Geometry: final body of the model. Coordinates: model frame, mm. Face numbers are marked on the shaded views. A direction names the side the tool comes from. Coordinates: 2 decimals unless noted, no trailing zeros. Loops run counter-clockwise (first coordinate to the right, second up) from the corner with the lowest first, then second, coordinate; pieces in that order, holes last. Notation, with made-up numbers: M -7.75,72.25 L 15.25,72.25 A18 ccw 15.25,83.25 Z; hole C 74.5,37.5 d2. An arc over 180 degrees is marked long. Write each question's results on one line, items separated by ' | '. Start each with the question number.
from build123d import *


with BuildPart() as part:
    # Sketch1 → Revolve3 (revolve)
    with BuildSketch(Plane.XY, mode=Mode.PRIVATE) as revolve3_sk:
        with BuildLine():
            Line((0, 0), (22.86, 0))
            Line((22.86, 0), (25.4, 2.54))
            Line((25.4, 2.54), (25.4, 8.89))
            Line((25.4, 8.89), (21.59, 12.7))
            Line((21.59, 12.7), (0, 12.7))
            Line((0, 12.7), (0, 11.43))
            Line((0, 11.43), (4.988818102, 8.549704526))
            ThreePointArc((4.988818102, 8.549704526), (6.258818102, 6.35), (4.988818102, 4.150295474))
            Line((4.988818102, 4.150295474), (0, 1.27))
            Line((0, 1.27), (0, 0))
        make_face()
    revolve(revolve3_sk.sketch.rotate(Axis((41.91, 0, 0), (0, 1, 0)), 270), axis=Axis((41.91, 0, 0), (0, 1, 0)))


solid = part.part
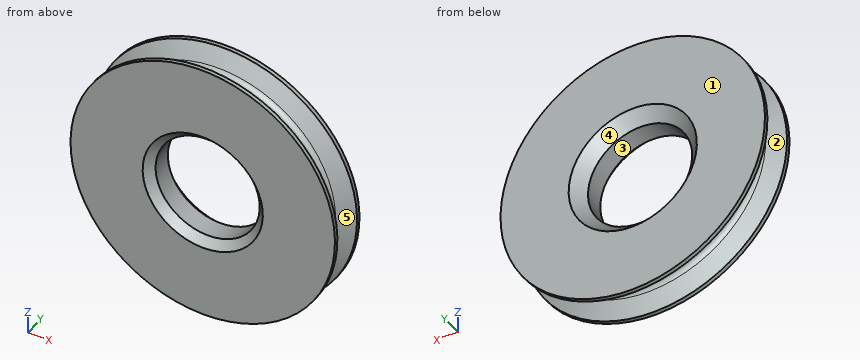
Item 1: Section C-C, the plane y = 7.5. Return loops of the section in (x, z).
Item 2: Contact query for flat-ended pins moving along their axis: P1, Ø1.5, axis at x = 32.5, y = 2.5, coming from the -Z side; P2, Ø4, axis at y = 5.5, z = 12.5, coming from the -X side. Output: stop coordinate, or through.
Item 3: Section A-A, the plane x = 41.91. Return loops of the section in (y, z).
Item 4: Pull-direction query (Z, two-part tool) for the marked faces 1, 2 and 3; classes: released by +Z, released by -Z, zero draft, split by the parting line, or undercut.
Item 5: Section B-B, the plane z = 0. Return loops of the section in (x, y), plus the area to 3 significant figures.
Item 6: Set-up query: the marked faces 4 and 5. Return all of +Z, -Z, +X, -X, +Y, -Y with unobstructed straight access to the full face (end or side cutting, diameter ignored); none if empty.
Item 7: Ray query, L1, parallel to X at y = 11, z = 1.5; L2, parallel to X at y = 5, z = 0; L3, parallel to Y at x = 27, z = -35. Return the intervals inside material, ascending. Write a range as [from, to].
Solutions:
1) outline: C 41.91,0 d71.85; hole C 41.91,0 d33.02
2) P1: stops at z = -40 | P2: stops at x = 5.91
3) outline: M 0,-41.91 L 1.27,-41.91 L 4.15,-36.92 A2.54 cw 8.55,-36.92 L 11.43,-41.91 L 12.7,-41.91 L 12.7,-20.32 L 8.89,-16.51 L 2.54,-16.51 L 0,-19.05 Z; M 0,19.05 L 2.54,16.51 L 8.89,16.51 L 12.7,20.32 L 12.7,41.91 L 11.43,41.91 L 8.55,36.92 A2.54 cw 4.15,36.92 L 1.27,41.91 L 0,41.91 Z
4) face 1: zero draft | face 2: split by the parting line | face 3: undercut
5) outline: M 0,0 L 22.86,0 L 25.4,2.54 L 25.4,8.89 L 21.59,12.7 L 0,12.7 L 0,11.43 L 4.99,8.55 A2.54 cw 4.99,4.15 L 0,1.27 Z; M 58.42,2.54 L 60.96,0 L 83.82,0 L 83.82,1.27 L 78.83,4.15 A2.54 cw 78.83,8.55 L 83.82,11.43 L 83.82,12.7 L 62.23,12.7 L 58.42,8.89 Z | area: 544 mm²
6) face 4: +Y | face 5: none
7) L1: x = [0.77, 23.35], [60.47, 83.05] | L2: x = [5.87, 25.4], [58.42, 77.95] | L3: y = [0, 3.5], [9.2, 12.7]
